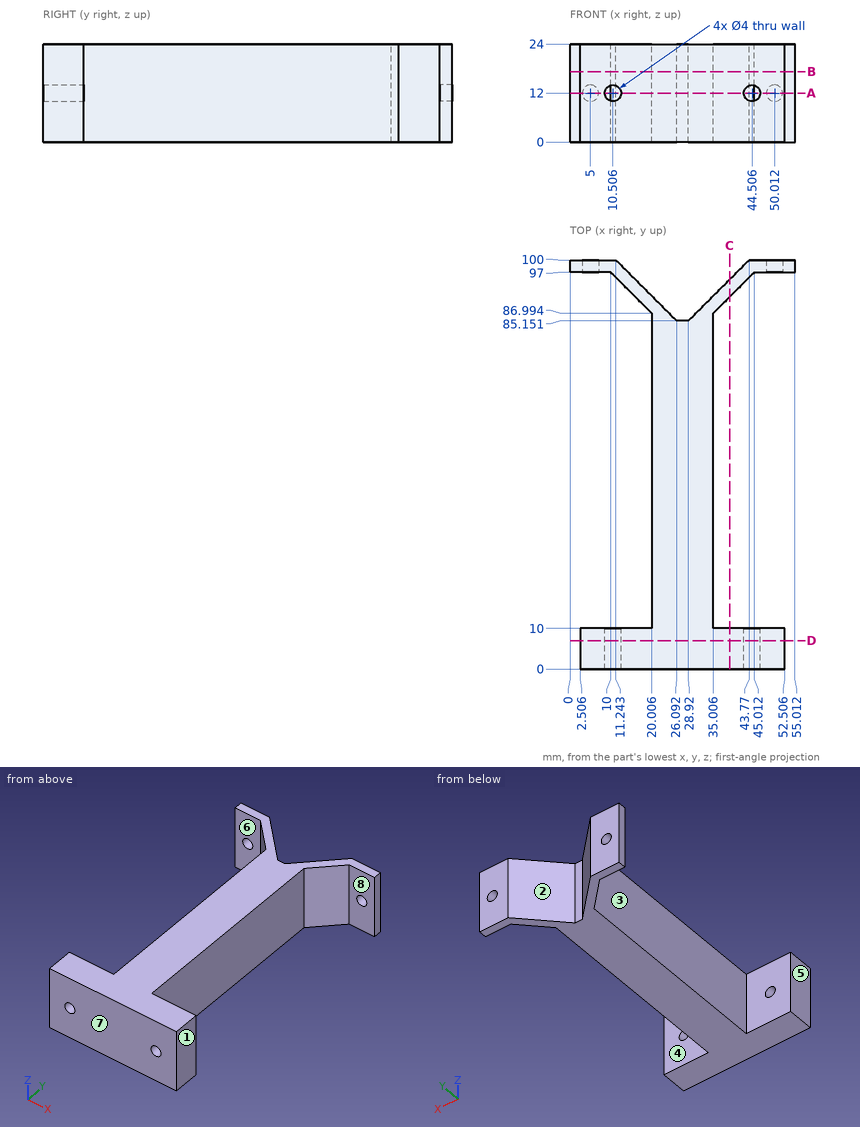
Input: dimensioned drawing with shaded views. Units: mm. Origin: part minimum x, y, z. A direction names the side the tool comes from. Coordinates: 2 decimals unless noted, no trailing zeros. Order: outer loops, then holes, each group sorted by start corner. A loop starts at its lowest first (then second) coordinate and runs counter-clockwise, first axis right, second up.
(1) Draft query along X for the marked faces 1, 2, 3 and 4. Return one class per face: pulls with the +X half, pulls with the -X half, needs draft (parallel to the pull), parting line crosses it, or undercut.
(2) Material intervals for probe 1 along X at (y, z) = (8, 12); probe 2 along Y at (x, z) = (45, 19.5); probe 3 along Z at (x, y) = (5, 98.8), sorted ascending.
(3) Section query B-B (z = 17.25). Return the cut outline in (x, y).
(4) Section query A-A (z = 12). State how many separate pieces and enclosed holes the cut face has, plus the area to 3 significant figures.
(5) First-contact query: pin 1 (8 mm diameter, centred on y = 39, z = 11, fed in from -X); pin 2 (5 mm diameter, centred on y = 4, z = 12, fed in from +X); pin 3 (8 mm diameter, centred on y = 4.5, z = 9.5, fed in from -X); pin 4 (6 mm diameter, centred on x = 41, y = 44, fed in from -Z). Flat tips, straight axial feed; report the tip coordinate or a pass-through.
(6) Access query for the marked faces 5, 6, 7 and 8. Directions: +Z, -Z, +X, -X, +Y, -Y. A direction counts if a zero-diameter tool reaches every point of the face in a straight line with its end or side. Return the directions, or none.
(7) Section query C-C (x = 39). Return the cut outline in (y, z).
(8) Section query D-D (y = 7). Return the cut outline in (x, z).
Solution:
1. face 1: pulls with the +X half
1. face 2: undercut
1. face 3: pulls with the -X half
1. face 4: needs draft
2. probe 1: x = 2.51 to 8.51, 12.51 to 42.51, 46.51 to 52.51
2. probe 2: y = 0 to 10, 96.99 to 100
2. probe 3: z = 0 to 10, 14 to 24
3. outline: (0, 97) - (10, 97) - (20.01, 86.99) - (20.01, 10) - (2.51, 10) - (2.51, 0) - (52.51, 0) - (52.51, 10) - (35.01, 10) - (35.01, 86.99) - (45.01, 97) - (55.01, 97) - (55.01, 100) - (43.77, 100) - (28.92, 85.15) - (26.09, 85.15) - (11.24, 100) - (0, 100) - close
4. separate pieces: 5
4. enclosed holes: 0
4. area: 1,700 mm2
5. pin 1: stops at x = 20.01
5. pin 2: stops at x = 52.51
5. pin 3: stops at x = 2.51
5. pin 4: passes through
6. face 5: +Z, -Z, -X, -Y
6. face 6: +Z, -Z, -X
6. face 7: +Z, -Z, +X, -X, -Y
6. face 8: +Z, -Z, +X
7. outline: (0, 0) - (10, 0) - (10, 24) - (0, 24) - close; (90.99, 0) - (95.23, 0) - (95.23, 24) - (90.99, 24) - close
8. outline: (2.51, 0) - (52.51, 0) - (52.51, 24) - (2.51, 24) - close; hole circle Ø4 at (10.51, 12); hole circle Ø4 at (44.51, 12)
